```python
from build123d import *

# Parameters (mm, degrees)
SKETCH_1_R      = 1.5
EXTRUDE_1_DEPTH = 4


with BuildPart() as part:
    # 草图1 → 凸台-拉伸1 (new body)
    with BuildSketch(Plane.XY):
        Polygon((0, 0), (0, 94), (-90, 104), (-103, 104), (-103, 84), (-93, 0), (-56.5, -16), (-36.5, -16), align=None)
        with Locations((-86.5, 15)):
            Circle(SKETCH_1_R, mode=Mode.SUBTRACT)
        with Locations(Location((-86.5, 5, 0), (0, 0, 180))):
            Circle(SKETCH_1_R, mode=Mode.SUBTRACT)
        with Locations((-6.5, 5)):
            Circle(SKETCH_1_R, mode=Mode.SUBTRACT)
        with Locations(Location((-6.5, 15, 0), (0, 0, 180))):
            Circle(SKETCH_1_R, mode=Mode.SUBTRACT)
        with Locations((-96.5, 99)):
            Circle(SKETCH_1_R, mode=Mode.SUBTRACT)
        with Locations((-96.5, 89)):
            Circle(SKETCH_1_R, mode=Mode.SUBTRACT)
        with Locations((-46.5, 14)):
            Circle(SKETCH_1_R, mode=Mode.SUBTRACT)
        with Locations((-46.5, 34)):
            Circle(SKETCH_1_R, mode=Mode.SUBTRACT)
        with Locations((-46.5, 54)):
            Circle(SKETCH_1_R, mode=Mode.SUBTRACT)
        with Locations((-46.5, 74)):
            Circle(SKETCH_1_R, mode=Mode.SUBTRACT)
        with Locations((-46.5, -6)):
            Circle(SKETCH_1_R, mode=Mode.SUBTRACT)
        with Locations((-25, 88)):
            Circle(SKETCH_1_R, mode=Mode.SUBTRACT)
        with Locations((-5, 88)):
            Circle(SKETCH_1_R, mode=Mode.SUBTRACT)
    extrude(amount=EXTRUDE_1_DEPTH)


solid = part.part
```
Could you check a few things on this model? Use its own coordinates, in mm. Give positions to 0.01 mm unless a question says otherwise; leave off trailing zeros. Loops run counter-clockwise (first coordinate to the right, second up) from the corner with the lowest first, then second, coordinate; pieces in that order, holes last. Notation, with made-up numbers: (80.5, -1.5) -> (131.5, -1.5) arc R7 ccw to (131.5, 7.5) -> close; hole circle Ø7 at (-28, 2). An arc over 180 degrees is marked (long way). Put each result on its own line as item: value.
(1) Imagine slicing it at C-C on z = 1.7. State how many separate pieces and enclosed holes the cut face has, plus the area to 3 significant figures.
Computed:
separate pieces: 1
enclosed holes: 13
area: 10,700 mm^2
(2) Thinking about a two-plate mould opening in Y: for faces 1 (the face through (-47.7, 53.1, 2)), 2 (the face through (-96, 104, 2)), 3 (the face through (-52, 45, 4)), which applies, pulls with the +Y half, pulls with the -Y half, needs draft (parallel to the pull), parting line crosses it, or undercut?
Computed:
face 1: undercut
face 2: pulls with the +Y half
face 3: needs draft
(3) Imagine slicing it at B-B on x = -46.5. Write out the boundary of the cut face in (y, z), plus the area to 3 significant figures.
Computed:
outline: (-16, 0) -> (-7.5, 0) -> (-7.5, 4) -> (-16, 4) -> close; (-4.5, 0) -> (12.5, 0) -> (12.5, 4) -> (-4.5, 4) -> close; (15.5, 0) -> (32.5, 0) -> (32.5, 4) -> (15.5, 4) -> close; (35.5, 0) -> (52.5, 0) -> (52.5, 4) -> (35.5, 4) -> close; (55.5, 0) -> (72.5, 0) -> (72.5, 4) -> (55.5, 4) -> close; (75.5, 0) -> (99.17, 0) -> (99.17, 4) -> (75.5, 4) -> close
area: 401 mm^2
(4) Please list where these lines run through material, in increasing order: probe 1 along Y at (x, z) = (-46.5, 1.35); probe 2 along X at (y, z) = (89, 3.1); probe 3 along X at (y, z) = (88, 2.95). Write a range as [from, to].
Computed:
probe 1: [-16, -7.5], [-4.5, 12.5], [15.5, 32.5], [35.5, 52.5], [55.5, 72.5], [75.5, 99.17]
probe 2: [-103, -98], [-95, -26.12], [-23.88, -6.12], [-3.88, 0]
probe 3: [-103, -97.62], [-95.38, -26.5], [-23.5, -6.5], [-3.5, 0]
(5) Imagine slicing it at A-A on x = -96.5. Write out the boundary of the cut face in (y, z).
Computed:
outline: (29.4, 0) -> (87.5, 0) -> (87.5, 4) -> (29.4, 4) -> close; (90.5, 0) -> (97.5, 0) -> (97.5, 4) -> (90.5, 4) -> close; (100.5, 0) -> (104, 0) -> (104, 4) -> (100.5, 4) -> close
(6) I'm going to push flat-ended pins straight in: pin 1 Ø2 at (x, z) = (-34.5, 3.5) entering from +Y; pin 2 Ø2 at (x, z) = (-29, 1.5) entering from -Y; pin 3 Ø1 at (x, z) = (-54.5, 2) entering from +Y. Where does each tip first touch, or does it pass through?
Computed:
pin 1: y = 97.94
pin 2: y = -13.15
pin 3: y = 100.11
(7) Imagine slicing it at D-D on y = 34. Write out the boundary of the cut face in (x, z), plus the area to 3 significant figures.
Computed:
outline: (-97.05, 0) -> (-48, 0) -> (-48, 4) -> (-97.05, 4) -> close; (-45, 0) -> (0, 0) -> (0, 4) -> (-45, 4) -> close
area: 376 mm^2
